Autodesk Inventor part; units mm, degrees
ref_plane "YZ Plane" through (0, 0, 0) normal (1, 0, 0) x (0, 1, 0)
ref_plane "XZ Plane" through (0, 0, 0) normal (0, 1, 0) x (-1, 0, 0)
ref_plane "XY Plane" through (0, 0, 0) normal (0, 0, 1) x (1, 0, 0)
sketch "Sketch2" plane through (0, 0, 0) normal (0, 1, 0) x (-1, 0, 0)
  line L0 (0, 0) -> (-285.75, 0)
  line L1 (-285.75, 0) -> (-285.75, 774.7)
  line L2 (-285.75, 774.7) -> (0, 774.7)
  line L3 (0, 774.7) -> (0, 692.15)
  line L4 (0, 692.15) -> (-203.2, 692.15)
  line L5 (-203.2, 692.15) -> (-203.2, 82.55)
  line L6 (-203.2, 82.55) -> (0, 82.55)
  line L7 (0, 82.55) -> (0, 0)
  dimension "d0" = 82.55
  dimension "d1" = 203.2
  dimension "d2" = 82.55
  dimension "d4" = 609.6
extrude "Extrusion1" add sketch "Sketch2" along normal blind 101.6
fillet "Fillet1" radius 25.4 6 edges at (285.75, 101.6, 387.35) (285.75, 0, 387.35) (142.875, 101.6, 0) (142.875, 101.6, 774.7) (142.875, 0, 774.7) (142.875, 0, 0)
properties part number "BumperRepresentation"
Read the model definition and answer for the solid it produces. Units are mm, in the model's axes. A direction names the side the tool comes from. Coordinates: 2 decimals unless noted, no trailing zeros. Order: outer loops, then holes, each group sorted by start corner. A loop starts at its lowest first (then second) coordinate and runs counter-clockwise, first axis right, second up. Notation, with made-up numbers: (39.25, 86.25) - (82.25, 86.25) arc R27 ccw to (82.25, 111.25) - close; hole circle Ø7 at (26, 34.5). An arc over 180 degrees is marked (long way). Answer as a JSON object with one key per item and string values. Group by question number.
Item 1: Section D-D (y = 55.5) is taken. Give the vertices of the cut face in (x, z), plus the area to 3 significant figures.
Item 2: The mould has two halves that part along Z. Classify faces 1 (the face through (285.75, 50, 382)), 2 (the face through (140.87, 7.24, 767.06)), 3 (the face through (103, 50, 82.55)): +Z half, -Z half, draft (parallel to the pull), parting line (faces both ways), or undercut.
Item 3: Section A-A (x = 145) is taken. Give the vertices of the cut face in (y, z), plus the area to 3 significant figures.
Item 4: Section C-C (y = 17) is taken. Give the vertices of the cut face in (x, z).
Item 5: Section B-B (z = 188) is taken. Give the vertices of the cut face in (x, y), plus the area to 3 significant figures.
Item 6: Flat-ended cylindrical pins translate along their axes: P1, Ø1.5, axis at x = 242, y = 80.5, coming from the +Z side; P2, Ø8, axis at y = 56.5, z = 298.5, coming from the -X side; P3, Ø5, axis at x = 137, y = 83.5, coming from the -Z side. Find the tip coordinate at first contact, or state that the pin passes through.
Item 7: Consider probe 1 along Z at (x, y) = (178.5, 45); probe 2 along X at (y, z) = (47.5, 496); probe 3 along X at (y, z) = (79, 53.5). Determine where each line is inside the solid, lowest interval first. Write a range as from..to.
Item 8: A tool of negligible diameter and unlimited length cuts with its end or side. For faces 4 (the face through (141, 50, 0)), 5 (the face through (203.2, 50, 392)), from which of +Z, -Z, +X, -X, +Y, -Y can it reach the whole face along a straight path? Write none if from no direction.
Results are:
{
 "1": {"outline": "(0, 0) - (285.75, 0) - (285.75, 774.7) - (0, 774.7) - (0, 692.15) - (203.2, 692.15) - (203.2, 82.55) - (0, 82.55) - close", "area": "97,500 mm^2"},
 "2": {"face 1": "draft", "face 2": "+Z half", "face 3": "undercut"},
 "3": {"outline": "(0, 25.4) arc R25.4 ccw to (25.4, 0) - (76.2, 0) arc R25.4 ccw to (101.6, 25.4) - (101.6, 82.55) - (0, 82.55) - close; (0, 692.15) - (101.6, 692.15) - (101.6, 749.3) arc R25.4 ccw to (76.2, 774.7) - (25.4, 774.7) arc R25.4 ccw to (0, 749.3) - close", "area": "16,200 mm^2"},
 "4": {"outline": "(0, 1.43) - (284.32, 1.43) - (284.32, 773.27) - (0, 773.27) - (0, 692.15) - (203.2, 692.15) - (203.2, 82.55) - (0, 82.55) - close"},
 "5": {"outline": "(203.2, 0) - (260.35, 0) arc R25.4 ccw to (285.75, 25.4) - (285.75, 76.2) arc R25.4 ccw to (260.35, 101.6) - (203.2, 101.6) - close", "area": "8,110 mm^2"},
 "6": {"P1": "stops at z = 774.45", "P2": "stops at x = 203.2", "P3": "stops at z = 0.46"},
 "7": {"probe 1": "z = 0..82.55, 692.15..774.7", "probe 2": "x = 203.2..285.75", "probe 3": "x = 0..285.6"},
 "8": {"face 4": "-Z, +X, -X, +Y, -Y", "face 5": "-X, +Y, -Y"}
}
